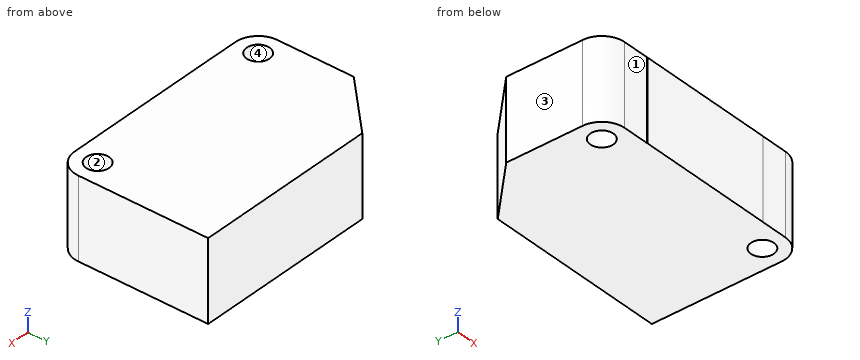
```python
from build123d import *

# Parameters (mm, degrees)
BOSS_EXTRU_1_DEPTH      = 10.5
ESQUISSE2_R             = 1.5
ENL_V_MAT_EXTRU_1_DEPTH = 39.356876828
CONG_1_R                = 3
ESQUISSE3_W             = 18
ESQUISSE3_H             = 10.5
BOSS_EXTRU_2_DEPTH      = 0.01


with BuildPart() as part:
    # Esquisse1 → Boss.-Extru.1 (new body)
    with BuildSketch(Plane.XY):
        Polygon((0, 0), (31, 0), (31, 20), (7, 20), (0, 13), align=None)
    extrude(amount=-BOSS_EXTRU_1_DEPTH)

    # Esquisse2 → Enlèv. mat.-Extru.1 (cut, through all)
    with BuildSketch(Plane.XY):
        with Locations((3, 3)):
            Circle(ESQUISSE2_R)
        with Locations((28, 3)):
            Circle(ESQUISSE2_R)
    extrude(amount=-ENL_V_MAT_EXTRU_1_DEPTH, mode=Mode.SUBTRACT)

    # Congé1
    cong_1_edges = [part.edges().sort_by_distance(p)[0] for p in [
        (31, 0, -5.25),
        (0, 0, -5.25),
    ]]
    fillet(cong_1_edges, radius=CONG_1_R)

    # Esquisse3 → Boss.-Extru.2 (add)
    with BuildSketch(Plane.XZ):
        with Locations((15.5, -5.25)):
            Rectangle(ESQUISSE3_W, ESQUISSE3_H)
    extrude(amount=BOSS_EXTRU_2_DEPTH)


solid = part.part
```
Can you work these out from the model? Positions are in its coordinate system, mm. Face numbers are marked on the shaded views. Coordinates: 2 decimals unless noted, no trailing zeros. Loops run counter-clockwise (first coordinate to the right, second up) from the corner with the lowest first, then second, coordinate; pieces in that order, holes last. Notation, with made-up numbers: (-37, 62.5) - (-2, 62.5) arc R28 ccw to (-2, 98.5) - close; hole circle Ø9 at (-16.75, 62.5). An arc over 180 degrees is marked (long way). Use a Markdown table: item, result.
Item 1: I want a section at C-C on x = 27.5. Please give me the cut outline in (y, z).
Numbers:
| item | result |
|---|---|
| outline | (0, -10.5) - (1.59, -10.5) - (1.59, 0) - (0, 0) - close; (4.41, -10.5) - (20, -10.5) - (20, 0) - (4.41, 0) - close |
Item 2: I want a section at A-A on x = 2. Please give me the cut outline in (y, z).
Numbers:
| item | result |
|---|---|
| outline | (0.17, -10.5) - (1.88, -10.5) - (1.88, 0) - (0.17, 0) - close; (4.12, -10.5) - (15, -10.5) - (15, 0) - (4.12, 0) - close |
Item 3: We'd pull the mould along Y, two halves only. Please class the marked faces 1, 2, 3 and 4: released by +Y, released by -Y, zero draft, split by the parting line, or undercut.
Numbers:
| item | result |
|---|---|
| face 1 | released by -Y |
| face 2 | undercut |
| face 3 | zero draft |
| face 4 | undercut |
Item 4: If I drill on probe 1 along Y at (x, z) = (28, -7); probe 2 along X at (y, z) = (2.5, -0.25); probe 3 along Y at (x, z) = (4, -5.25), over which ranges is the centre line in solid material (lowest first)? Write a range as from..to.
Numbers:
| item | result |
|---|---|
| probe 1 | y = 0..1.5, 4.5..20 |
| probe 2 | x = 0.04..1.59, 4.41..26.59, 29.41..30.96 |
| probe 3 | y = 0..1.88, 4.12..17 |
Item 5: I want a section at B-B on z = -1.25. Give the number of separate pieces and of enclosed holes in the cut face, and give its area (3 significant figures).
Numbers:
| item | result |
|---|---|
| separate pieces | 1 |
| enclosed holes | 2 |
| area | 578 mm2 |
Item 6: Will these pins go through, and if not, where does the flat tip stop? pin 1 (2 mm diameter, centred on y = 16, z = -4.5, fed in from -X); pin 2 (1.8 mm diameter, centred on x = 4, z = -6.5, fed in from -Y); pin 3 (2.5 mm diameter, centred on x = 3, y = 3, fed in from -Z).
Numbers:
| item | result |
|---|---|
| pin 1 | stops at x = 2 |
| pin 2 | stops at y = 0 |
| pin 3 | passes through |
